Could you check a few things on this model? Use its own coordinates, in mm. Coordinates: 2 decimals unless noted, no trailing zeros. Loops run counter-clockwise (first coordinate to the right, second up) from the corner with the lowest first, then second, coordinate; pieces in that order, holes last. Notation, with made-up numbers: (77.5, 17) - (96.5, 17) arc R22 ccw to (96.5, 36) - close; hole circle Ø2 at (81, -15). An arc over 180 degrees is marked (long way). One line per question, with ' | ' between items. Start each with the question number.
1. I'm going to push a flat-ended pin straight in: P1, Ø6, axis at x = 150, z = 15, coming from the +Y side. Where does the tip first touch, or does it pass through?
2. I want a section at A-A, the plane z = 126.5. Write out the boundary of the cut face in (x, y).
3. Please list where these lines run through material, in increasing order: L1, parallel to X at y = -1.5, z = 215; L2, parallel to Z at x = 15, y = -2.1; L3, parallel to X at y = -4.5, z = 128. Write a range as [from, to].
from build123d import *

# Parameters (mm, degrees)
F0_W     = 520
F0_H     = 330
F0_R     = 3.25
F1_DEPTH = 5
F2_R     = 5


with BuildPart() as f1:
    # F0 (on Front) → F1 (new body)
    with BuildSketch(Plane.XZ):
        with Locations((260, 165)):
            Rectangle(F0_W, F0_H)
        with Locations((15, 15)):
            Circle(F0_R, mode=Mode.SUBTRACT)
        with Locations((150, 15)):
            Circle(F0_R, mode=Mode.SUBTRACT)
        with Locations((15, 115)):
            Circle(F0_R, mode=Mode.SUBTRACT)
        with BuildLine():
            Line((217.55, 106), (217.55, 146))
            ThreePointArc((217.55, 146), (220.8, 149.25), (224.05, 146))
            Line((224.05, 146), (224.05, 106))
            ThreePointArc((224.05, 106), (220.8, 102.75), (217.55, 106))
        make_face(mode=Mode.SUBTRACT)
        with Locations((370, 15)):
            Circle(F0_R, mode=Mode.SUBTRACT)
        with BuildLine():
            Line((256.75, 40), (256.75, 80))
            ThreePointArc((256.75, 80), (260, 83.25), (263.25, 80))
            Line((263.25, 80), (263.25, 40))
            ThreePointArc((263.25, 40), (260, 36.75), (256.75, 40))
        make_face(mode=Mode.SUBTRACT)
        with Locations((505, 15)):
            Circle(F0_R, mode=Mode.SUBTRACT)
        with BuildLine():
            Line((295.95, 106), (295.95, 146))
            ThreePointArc((295.95, 146), (299.2, 149.25), (302.45, 146))
            Line((302.45, 146), (302.45, 106))
            ThreePointArc((302.45, 106), (299.2, 102.75), (295.95, 106))
        make_face(mode=Mode.SUBTRACT)
        with Locations((505, 115)):
            Circle(F0_R, mode=Mode.SUBTRACT)
        with Locations((15, 215)):
            Circle(F0_R, mode=Mode.SUBTRACT)
        with Locations((15, 315)):
            Circle(F0_R, mode=Mode.SUBTRACT)
        with Locations((505, 215)):
            Circle(F0_R, mode=Mode.SUBTRACT)
        with Locations((505, 315)):
            Circle(F0_R, mode=Mode.SUBTRACT)
    extrude(amount=F1_DEPTH)

    # F2
    f2_edges = [f1.edges().sort_by_distance(p)[0] for p in [
        (520, -2.5, 330),
        (520, -2.5, 0),
        (0, -2.5, 0),
        (0, -2.5, 330),
    ]]
    fillet(f2_edges, radius=F2_R)


solid = f1.part
Results are:
1) P1: passes through
2) outline: (0, -5) - (217.55, -5) - (217.55, 0) - (0, 0) - close; (224.05, -5) - (295.95, -5) - (295.95, 0) - (224.05, 0) - close; (302.45, -5) - (520, -5) - (520, 0) - (302.45, 0) - close
3) L1: x = [0, 11.75], [18.25, 501.75], [508.25, 520] | L2: z = [0, 11.75], [18.25, 111.75], [118.25, 211.75], [218.25, 311.75], [318.25, 330] | L3: x = [0, 217.55], [224.05, 295.95], [302.45, 520]
